```python
from build123d import *

# Parameters (mm, degrees)
SKETCH1_R                                           = 47.5
SKETCH1_R_2                                         = 35
BOSS_EXTRUDE1_DEPTH                                 = 9.5
SKETCH2_R                                           = 2.25
CUT_EXTRUDE1_DEPTH                                  = 10
CSK_FOR_M4_COUNTERSUNK_FLAT_HEAD_SCREW1_D           = 4.5
CSK_FOR_M4_COUNTERSUNK_FLAT_HEAD_SCREW1_CSINK_D     = 9.4
CSK_FOR_M4_COUNTERSUNK_FLAT_HEAD_SCREW1_CSINK_ANGLE = 90


with BuildPart() as part:
    # Sketch1 → Boss-Extrude1 (new body)
    with BuildSketch(Plane(origin=(0, 0, 0), x_dir=(1, 0, 0), z_dir=(0, 1, 0))):
        with Locations(Location((0, 0, 0), (0, 0, 270))):
            Circle(SKETCH1_R)
        with Locations(Location((0, 0, 0), (0, 0, 270))):
            Circle(SKETCH1_R_2, mode=Mode.SUBTRACT)
    extrude(amount=BOSS_EXTRUDE1_DEPTH)

    # Sketch2 → Cut-Extrude1 (cut)
    with BuildSketch(Plane(origin=(0, 9.5, 0), x_dir=(1, 0, 0), z_dir=(0, 1, 0))):
        with Locations(Location((0, 41.25, 0), (0, 0, 270))):
            Circle(SKETCH2_R)
        with Locations(Location((41.25, 0, 0), (0, 0, 270))):
            Circle(SKETCH2_R)
        with Locations(Location((0, -41.25, 0), (0, 0, 270))):
            Circle(SKETCH2_R)
        with Locations(Location((-41.25, 0, 0), (0, 0, 270))):
            Circle(SKETCH2_R)
    extrude(amount=-CUT_EXTRUDE1_DEPTH, mode=Mode.SUBTRACT)

    # CSK for M4 Countersunk Flat Head Screw1 (through all)
    with Locations(Plane(origin=(0, 9.5, 41.25), x_dir=(0, 0, 1), z_dir=(0, 1, 0))):
        with Locations((0, 0), (-41.25, 41.25), (-82.5, 0), (-41.25, -41.25)):
            CounterSinkHole(CSK_FOR_M4_COUNTERSUNK_FLAT_HEAD_SCREW1_D / 2, CSK_FOR_M4_COUNTERSUNK_FLAT_HEAD_SCREW1_CSINK_D / 2, counter_sink_angle=CSK_FOR_M4_COUNTERSUNK_FLAT_HEAD_SCREW1_CSINK_ANGLE)


solid = part.part
```
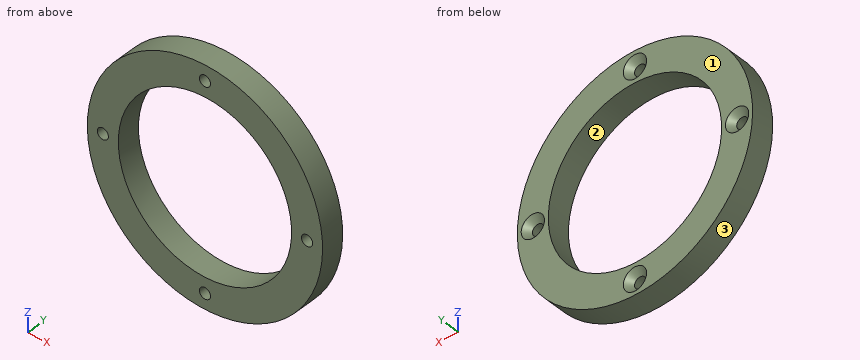
Part model, mm, in its own coordinate system. Face numbers are marked on the shaded views. Coordinates: 2 decimals unless noted, no trailing zeros. Write each loop counter-clockwise with the first axis right and the second up, starting at its lowest first coordinate (ties: lowest second). Pieces come first, ordered by that corner, then holes.
Item 1: Slice it at A-A (x = 0). Write the cut outline in (y, z), and give its area (3 significant figures).
Item 2: Probe line 1 (X direction, y = 3.75, z = 0); line 2 (X direction, y = 8, z = 24.5) (3 decimals); line 3 (X direction, y = 7.75, z = -41). List the from-to ranges inside material, lowest first.
Item 3: Mould opens along Z. For the marked faces 1, 2 and 3 say: released by +Z, released by -Z, zero draft, split by the parting line, or undercut.
Item 4: Slice it at B-B (z = 0). Write the cut outline in (x, y).
Item 5: Slice it at C-C (z = -11.5). Write the cut outline in (x, y).
Item 6: Slice it at D-D (y = 1.5). Write the cut outline in (x, z).
Item 7: Pin check, flat tips, straight feed: pin 1 (3.5 mm diameter, centred on x = -41.25, z = 0, fed in from +Y); pin 2 (2 mm diameter, centred on x = 38, y = 3, fed in from +Z); pin 3 (6 mm diameter, centred on x = 41.25, z = 0, fed in from +Y); pin 4 (2 mm diameter, centred on y = 1.5, z = -35.5, fed in from +X). Stop position of each tip, or through.
Results found:
1. outline: (0, -47.5) - (9.5, -47.5) - (9.5, -45.95) - (7.05, -43.5) - (0, -43.5) - close; (0, -39) - (7.05, -39) - (9.5, -36.55) - (9.5, -35) - (0, -35) - close; (0, 35) - (9.5, 35) - (9.5, 36.55) - (7.05, 39) - (0, 39) - close; (0, 43.5) - (7.05, 43.5) - (9.5, 45.95) - (9.5, 47.5) - (0, 47.5) - close
1. area: 140 mm2
2. line 1: x = -47.5 to -43.5, -39 to -35, 35 to 39, 43.5 to 47.5
2. line 2: x = -40.694 to -24.995, 24.995 to 40.694
2. line 3: x = -23.98 to -2.94, 2.94 to 23.98
3. face 1: zero draft
3. face 2: undercut
3. face 3: split by the parting line
4. outline: (-47.5, 0) - (-43.5, 0) - (-43.5, 7.05) - (-45.95, 9.5) - (-47.5, 9.5) - close; (-39, 0) - (-35, 0) - (-35, 9.5) - (-36.55, 9.5) - (-39, 7.05) - close; (35, 0) - (39, 0) - (39, 7.05) - (36.55, 9.5) - (35, 9.5) - close; (43.5, 0) - (47.5, 0) - (47.5, 9.5) - (45.95, 9.5) - (43.5, 7.05) - close
5. outline: (-46.09, 0) - (-33.06, 0) - (-33.06, 9.5) - (-46.09, 9.5) - close; (33.06, 0) - (46.09, 0) - (46.09, 9.5) - (33.06, 9.5) - close
6. outline: circle Ø95 at (0, 0); hole circle Ø4.5 at (-41.25, 0); hole circle Ø70 at (0, 0); hole circle Ø4.5 at (0, -41.25); hole circle Ø4.5 at (0, 41.25); hole circle Ø4.5 at (41.25, 0)
7. pin 1: passes through
7. pin 2: stops at z = 29.79
7. pin 3: stops at y = 7.8
7. pin 4: stops at x = 32.65
